from build123d import *

# Parameters (mm, degrees)
SKETCH1_R           = 5
SKETCH1_R_2         = 100
BOSS_EXTRUDE1_DEPTH = 3


with BuildPart() as part:
    # Sketch1 → Boss-Extrude1 (new body)
    with BuildSketch(Plane.XY):
        with BuildLine():
            Line((-56.262313577, -154.579436119), (-51.538403725, -156.217934123))
            Line((-51.538403725, -156.217934123), (-54.671437386, -165.714465072))
            ThreePointArc((-54.671437386, -165.714465072), (-46.10465637, -168.299170114), (-37.416640882, -170.441324171))
            ThreePointArc((-37.416640882, -170.441324171), (-27.888102395, -167.417194297), (-25.739334079, -157.653936545))
            ThreePointArc((-25.739334079, -157.653936545), (0, -122.5), (25.739334079, -157.653936545))
            ThreePointArc((25.739334079, -157.653936545), (27.888102395, -167.417194297), (37.416640882, -170.441324171))
            ThreePointArc((37.416640882, -170.441324171), (48.657069904, -167.579054623), (59.68251501, -163.976362327))
            Line((59.68251501, -163.976362327), (56.262313577, -154.579436119))
            Line((56.262313577, -154.579436119), (60.934244684, -152.798127687))
            Line((60.934244684, -152.798127687), (64.638454088, -162.086767668))
            ThreePointArc((64.638454088, -162.086767668), (125.251113016, -121.500653037), (163.976362327, -59.68251501))
            Line((163.976362327, -59.68251501), (154.579436119, -56.262313577))
            Line((154.579436119, -56.262313577), (156.217934123, -51.538403725))
            Line((156.217934123, -51.538403725), (165.714465072, -54.671437386))
            ThreePointArc((165.714465072, -54.671437386), (168.299170114, -46.10465637), (170.441324171, -37.416640882))
            ThreePointArc((170.441324171, -37.416640882), (167.417194297, -27.888102395), (157.653936545, -25.739334079))
            ThreePointArc((157.653936545, -25.739334079), (122.5, 0), (157.653936545, 25.739334079))
            ThreePointArc((157.653936545, 25.739334079), (167.417194297, 27.888102395), (170.441324171, 37.416640882))
            ThreePointArc((170.441324171, 37.416640882), (167.579054623, 48.657069904), (163.976362327, 59.68251501))
            Line((163.976362327, 59.68251501), (154.579436119, 56.262313577))
            Line((154.579436119, 56.262313577), (152.798127687, 60.934244684))
            Line((152.798127687, 60.934244684), (162.086767668, 64.638454088))
            ThreePointArc((162.086767668, 64.638454088), (121.500653037, 125.251113016), (59.68251501, 163.976362327))
            Line((59.68251501, 163.976362327), (56.262313577, 154.579436119))
            Line((56.262313577, 154.579436119), (51.538403725, 156.217934123))
            Line((51.538403725, 156.217934123), (54.671437386, 165.714465072))
            ThreePointArc((54.671437386, 165.714465072), (46.10465637, 168.299170114), (37.416640882, 170.441324171))
            ThreePointArc((37.416640882, 170.441324171), (27.888102395, 167.417194297), (25.739334079, 157.653936545))
            ThreePointArc((25.739334079, 157.653936545), (0, 122.5), (-25.739334079, 157.653936545))
            ThreePointArc((-25.739334079, 157.653936545), (-27.888102395, 167.417194297), (-37.416640882, 170.441324171))
            ThreePointArc((-37.416640882, 170.441324171), (-48.657069904, 167.579054623), (-59.68251501, 163.976362327))
            Line((-59.68251501, 163.976362327), (-56.262313577, 154.579436119))
            Line((-56.262313577, 154.579436119), (-60.934244684, 152.798127687))
            Line((-60.934244684, 152.798127687), (-64.638454088, 162.086767668))
            ThreePointArc((-64.638454088, 162.086767668), (-125.251113016, 121.500653037), (-163.976362327, 59.68251501))
            Line((-163.976362327, 59.68251501), (-154.579436119, 56.262313577))
            Line((-154.579436119, 56.262313577), (-156.217934123, 51.538403725))
            Line((-156.217934123, 51.538403725), (-165.714465072, 54.671437386))
            ThreePointArc((-165.714465072, 54.671437386), (-168.299170114, 46.10465637), (-170.441324171, 37.416640882))
            ThreePointArc((-170.441324171, 37.416640882), (-167.417194297, 27.888102395), (-157.653936545, 25.739334079))
            ThreePointArc((-157.653936545, 25.739334079), (-122.5, 0), (-157.653936545, -25.739334079))
            ThreePointArc((-157.653936545, -25.739334079), (-167.417194297, -27.888102395), (-170.441324171, -37.416640882))
            ThreePointArc((-170.441324171, -37.416640882), (-167.579054623, -48.657069904), (-163.976362327, -59.68251501))
            Line((-163.976362327, -59.68251501), (-154.579436119, -56.262313577))
            Line((-154.579436119, -56.262313577), (-152.798127687, -60.934244684))
            Line((-152.798127687, -60.934244684), (-162.086767668, -64.638454088))
            ThreePointArc((-162.086767668, -64.638454088), (-121.500653037, -125.251113016), (-59.68251501, -163.976362327))
            Line((-59.68251501, -163.976362327), (-56.262313577, -154.579436119))
        make_face()
        with Locations((121.873399663, -52.131018514)):
            Circle(SKETCH1_R, mode=Mode.SUBTRACT)
        with Locations((58.775444452, 116.257983948)):
            Circle(SKETCH1_R, mode=Mode.SUBTRACT)
        with Locations((-124.289525039, -46.039349088)):
            Circle(SKETCH1_R, mode=Mode.SUBTRACT)
        Circle(SKETCH1_R_2, mode=Mode.SUBTRACT)
    extrude(amount=BOSS_EXTRUDE1_DEPTH)


solid = part.part
Verification items for the finished model (mm, model axes). Coordinates: 2 decimals unless noted, no trailing zeros. Write each loop counter-clockwise with the first axis right and the second up, starting at its lowest first coordinate (ties: lowest second). Pieces come first, ordered by that corner, then holes. Notation, with made-up numbers: M 62.5,56 L 66.5,56 A29 ccw 66.5,86 Z; hole C -24,23.25 d8. An arc over 180 degrees is marked long. Use a Markdown table: item, result.
Q1. Go/stop test with flat-tipped pins: P1, Ø16, axis at x = 58.78, y = 116.26, coming from the +Z side; P2, Ø1, axis at x = 22, z = 1, coming from the +Y side; P3, Ø1.5, axis at x = -133.5, z = 0.5, coming from the -Y side; P4, Ø1, axis at x = 70.5, z = 1.5, coming from the -Y side. Record where each tip stops, or that it passes through.
Reply:
| item | result |
|---|---|
| P1 | stops at z = 3 |
| P2 | stops at y = 134.58 |
| P3 | stops at y = -113.26 |
| P4 | stops at y = -159.84 |
Q2. Draft check along Y on faces 1 (the face through (-78, 78, 3)), 2 (the face through (124.53, -122.24, 1.48)), 3 (the face through (55.09, 119.637, 1.479)), 4 (the face through (-167.31, -27.79, 1.48)). Enter one of: +Y half, -Y half, draft (parallel to the pull), parting line (faces both ways), or undercut.
Reply:
| item | result |
|---|---|
| face 1 | draft |
| face 2 | -Y half |
| face 3 | undercut |
| face 4 | undercut |
Q3. Sectioned sample at B-B, the plane x = -91. Record the boundary of the cut face in (y, z), plus the area to 3 significant figures.
Reply:
| item | result |
|---|---|
| outline | M -148.89,0 L -41.46,0 L -41.46,3 L -148.89,3 Z; M 41.46,0 L 148.89,0 L 148.89,3 L 41.46,3 Z |
| area | 645 mm² |
Q4. Sectioned sample at C-C, the plane z = 1. Count the separate pieces of the cut face and the enclosed holes in it, plus the area to 3 significant figures.
Reply:
| item | result |
|---|---|
| separate pieces | 1 |
| enclosed holes | 4 |
| area | 53,700 mm² |
Q5. Sectioned sample at A-A, the plane y = -127.5. Record the boundary of the cut face in (x, z), plus the area to 3 significant figures.
Reply:
| item | result |
|---|---|
| outline | M -119.14,0 L -15.65,0 L -15.65,3 L -119.14,3 Z; M 15.65,0 L 119.14,0 L 119.14,3 L 15.65,3 Z |
| area | 621 mm² |
Q6. Thickness scan on line 1 (Y direction, x = -28, z = 0.8); line 2 (Y direction, x = -132.5, z = 1.3); line 3 (X direction, y = -41, z = 1.35) (3 decimals). Record the ranges inside material, lowest first.
Reply:
| item | result |
|---|---|
| line 1 | y = -167.54 to -96, 96 to 167.54 |
| line 2 | y = -113.55 to -20.98, 20.98 to 113.55 |
| line 3 | x = -169.615 to -91.209, 91.209 to 169.615 |
